from build123d import *

# Parameters (mm, degrees)
F0_R     = 228.6
F0_W     = 38.1
F0_H     = 88.9
F1_DEPTH = 19.05


with BuildPart() as f1:
    # F0 (on Front) → F1 (new body, symmetric)
    with BuildSketch(Plane.XZ):
        Circle(F0_R)
        Rectangle(F0_W, F0_H, mode=Mode.SUBTRACT)
    extrude(amount=F1_DEPTH, both=True)


solid = f1.part
The listing builds one solid part. Answer for the finished solid, in the listing's coordinates (mm). A direction names the side the tool comes from. Round coordinates to 2 decimals unless told otherwise and drop trailing zeros. Write each loop counter-clockwise with the first axis right and the second up, starting at its lowest first coordinate (ties: lowest second). Pieces come first, ordered by that corner, then holes. Notation, with made-up numbers: M 62,-28 L 96,-28 A35 cw 96,10 Z; hole C -19.75,34 d9. An arc over 180 degrees is marked long. Write each question's results on one line, items separated by ' | '. Start each with the question number.
Item 1: Straight lines are drawn through the part: L1, parallel to X at y = -5, z = -1.5; L2, parallel to X at y = 8.5, z = 13; L3, parallel to Z at x = -204, y = -14. For each, find the intervals that lie inside material, in ascending order. Write a range as [from, to].
Item 2: A cutting plane is placed at A-A on z = 0. Write down the section's boundary in (x, y).
Item 3: A cutting plane is placed at C-C on y = -2. Write down the section's boundary in (x, z).
Item 4: For a pull along X with two mould halves and no side action, classify faces 3 (the face through (19.05, 0, -1)), 4 (the face through (-228.38, -0.27, 10.05)), 5 (the face through (-3, -19.05, -48)) as pulls with the +X half, pulls with the -X half, needs draft (parallel to the pull), parting line crosses it, or undercut.
Item 5: A cutting plane is placed at B-B on x = 0. Write down the section's boundary in (y, z).
Item 6: For faces 1 (the face through (0, 0, 44.45)), 2 (the face through (-3, 19.05, -48)), determine the directions among +Z, -Z, +X, -X, +Y, -Y from which every point of the face is accessible in a straight line to the end or side of a thin tool.
Item 7: Flat-ended cylindrical pins translate along their axes: pin 1 Ø1.5 at (x, y) = (-80, -7) entering from -Z; pin 2 Ø8 at (x, y) = (-176.5, 12.5) entering from +Z; pin 3 Ø19 at (y, z) = (-5.5, 7.5) entering from +X; pin 4 Ø4 at (y, z) = (6.5, -41.5) entering from +X. Find the tip coordinate at first contact, or state that the pin passes through.
Item 8: A cutting plane is placed at D-D on x = 139. Write down the section's boundary in (y, z).
Check sheet entries:
1) L1: [-228.6, -19.05], [19.05, 228.6] | L2: [-228.23, -19.05], [19.05, 228.23] | L3: [-103.16, 103.16]
2) outline: M -228.6,-19.05 L -19.05,-19.05 L -19.05,19.05 L -228.6,19.05 Z; M 19.05,-19.05 L 228.6,-19.05 L 228.6,19.05 L 19.05,19.05 Z
3) outline: C 0,0 d457.2; hole M -19.05,-44.45 L 19.05,-44.45 L 19.05,44.45 L -19.05,44.45 Z
4) face 3: undercut | face 4: parting line crosses it | face 5: needs draft
5) outline: M -19.05,-228.6 L 19.05,-228.6 L 19.05,-44.45 L -19.05,-44.45 Z; M -19.05,44.45 L 19.05,44.45 L 19.05,228.6 L -19.05,228.6 Z
6) face 1: +Y, -Y | face 2: +Z, -Z, +X, -X, +Y
7) pin 1: z = -214.42 | pin 2: z = 150.01 | pin 3: x = 228.6 | pin 4: x = 225.16
8) outline: M -19.05,-181.49 L 19.05,-181.49 L 19.05,181.49 L -19.05,181.49 Z
